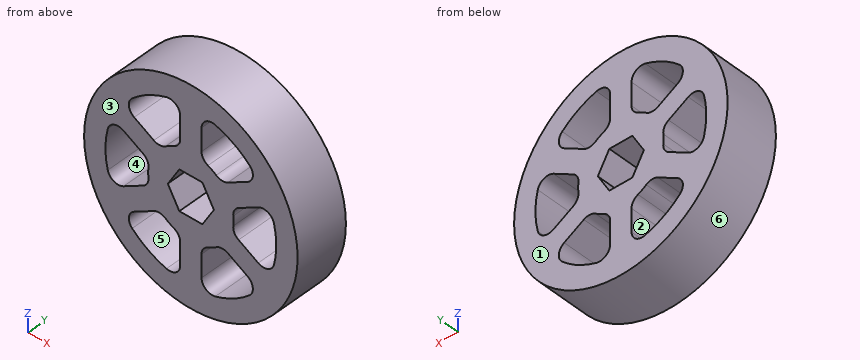
Autodesk Inventor part; units mm, degrees
ref_plane "YZ Plane" through (0, 0, 0) normal (1, 0, 0) x (0, 1, 0)
ref_plane "XZ Plane" through (0, 0, 0) normal (0, 1, 0) x (-1, 0, 0)
ref_plane "XY Plane" through (0, 0, 0) normal (0, 0, 1) x (1, 0, 0)
sketch "Sketch1" plane through (0, 0, 0) normal (0, 1, 0) x (-1, 0, 0)
  circle A0 centre (0, 0) radius 25.4
  line L0 (-2.7424, 4.75) -> (2.7424, 4.75)
  line L1 (2.7424, 4.75) -> (5.4848, 0)
  line L2 (5.4848, 0) -> (2.7424, -4.75)
  line L3 (2.7424, -4.75) -> (-2.7424, -4.75)
  line L4 (-2.7424, -4.75) -> (-5.4848, 0)
  line L5 (-5.4848, 0) -> (-2.7424, 4.75)
  line L6 (2.54, -9.8374) -> (2.54, -20.1606)
  line L7 (-2.54, -9.8374) -> (-2.54, -20.1606)
  line L8 (0, -11.1125) -> (0, -22.225) construction
  line L9 (9.7894, -2.719) -> (18.7296, -7.8806)
  line L10 (7.2494, -7.1184) -> (16.1896, -12.28)
  line L11 (7.2494, 7.1184) -> (16.1896, 12.28)
  line L12 (9.7894, 2.719) -> (18.7296, 7.8806)
  line L13 (-2.54, 9.8374) -> (-2.54, 20.1606)
  line L14 (2.54, 9.8374) -> (2.54, 20.1606)
  line L15 (-9.7894, 2.719) -> (-18.7296, 7.8806)
  line L16 (-7.2494, 7.1184) -> (-16.1896, 12.28)
  line L17 (-7.2494, -7.1184) -> (-16.1896, -12.28)
  line L18 (-9.7894, -2.719) -> (-18.7296, -7.8806)
  arc A1 (9.7894, -2.719) -> (9.7894, 2.719) centre (0, 0) ccw
  arc A2 (7.2494, 7.1184) -> (2.54, 9.8374) centre (0, 0) ccw
  arc A3 (-2.54, 9.8374) -> (-7.2494, 7.1184) centre (0, 0) ccw
  arc A4 (-9.7894, 2.719) -> (-9.7894, -2.719) centre (0, 0) ccw
  arc A5 (-16.1896, -12.28) -> (-2.54, -20.1606) centre (0, 0) ccw
  arc A6 (2.54, -20.1606) -> (16.1896, -12.28) centre (0, 0) ccw
  arc A7 (18.7296, -7.8806) -> (18.7296, 7.8806) centre (0, 0) ccw
  arc A8 (16.1896, 12.28) -> (2.54, 20.1606) centre (0, 0) ccw
  arc A9 (-2.54, 20.1606) -> (-16.1896, 12.28) centre (0, 0) ccw
  arc A10 (-18.7296, 7.8806) -> (-18.7296, -7.8806) centre (0, 0) ccw
  arc A11 (-7.2494, -7.1184) -> (-2.54, -9.8374) centre (0, 0) ccw
  arc A12 (2.54, -9.8374) -> (7.2494, -7.1184) centre (0, 0) ccw
  dimension "d1" = 9.5
  dimension "d4" = 5.08
  dimension "d7" = 360
  dimension "d9" = 20.32
  dimension "d10" = 10.16
  dimension "d11" = 25.4
extrude "Extrusion1" add sketch "Sketch1" along normal blind 12.7
fillet "Fillet1" radius 2.54 4 edges at (16.1896, 6.35, 12.28) (7.2494, 6.35, 7.1184) (2.54, 6.35, 9.8374) (2.54, 6.35, 20.1606)
pattern_circular "Circular Pattern1" count 6 over 360 about axis through (0, 0, 0) along (0, 1, 0) of "Fillet1"
properties part number "2in mould"
Part model, mm, in its own coordinate system. Face numbers are marked on the shaded views. A direction names the side the tool comes from. Coordinates: 2 decimals unless noted, no trailing zeros. Loops run counter-clockwise (first coordinate to the right, second up) from the corner with the lowest first, then second, coordinate; pieces in that order, holes last. Notation, with made-up numbers: (34.5, 42) -> (47.5, 42) arc R26 cw to (47.5, 67) -> close; hole circle Ø11 at (66, 28). An arc over 180 degrees is marked (long way). Use a Markdown table: item, result. Add a question column.
Item 1: Band-saw the part on D-D on x = -7.5. Write the cut outline in (y, z).
Item 2: Band-saw the part on B-B on z = -5.5. Write the cut outline in (x, y).
Item 3: Pull direction X, two halves, no side cores. Call the marked faces 3, 4, 5 and 6: +X half, -X half, draft (parallel to the pull), parting line (faces both ways), or undercut.
Item 4: Probe probe 1 along Z at (x, y) = (-11, 3.25); probe 2 along X at (y, z) = (2.5, 15); probe 3 along Z at (x, y) = (-11.5, 1). List the from-to ranges inside material, lowest first.
Item 5: Band-saw the part on A-A on x = 0. Write the cut outline in (y, z).
Item 6: Band-saw the part on C-C on y = 3.5. Give the number of separate pieces and of enclosed holes in the cut face, plus the area to 3 significant figures.
Item 7: Flat gauge pins, fed straight in: P1, Ø4.5, axis at x = 0, y = 8.5, coming from the +Z side; P2, Ø2.5, axis at y = 4.5, z = -14.5, coming from the -X side; P3, Ø1.5, axis at y = 7.5, z = 19, coming from the +X side. Where does each tip first touch, or does it go through?
Item 8: Which spindle directions (+Z, -Z, +X, -X, +Y, -Y) get a long thin tool onto all of the face, cutting with end or side? Do the marked faces 1 and 2. Say none if no direction does.
Geometry says:
| question | item | result |
|---|---|---|
| 1 | outline | (0, -24.27) -> (12.7, -24.27) -> (12.7, -18.89) -> (0, -18.89) -> close; (0, -7.68) -> (12.7, -7.68) -> (12.7, 7.68) -> (0, 7.68) -> close; (0, 18.89) -> (12.7, 18.89) -> (12.7, 24.27) -> (0, 24.27) -> close |
| 2 | outline | (-24.8, 0) -> (-19.43, 0) -> (-19.43, 12.7) -> (-24.8, 12.7) -> close; (-14.61, 0) -> (14.61, 0) -> (14.61, 12.7) -> (-14.61, 12.7) -> close; (19.43, 0) -> (24.8, 0) -> (24.8, 12.7) -> (19.43, 12.7) -> close |
| 3 | face 3 | draft |
| 3 | face 4 | undercut |
| 3 | face 5 | undercut |
| 3 | face 6 | parting line |
| 4 | probe 1 | -22.89 to -17.09, -9.28 to -3.38, 3.38 to 9.28, 17.09 to 22.89 |
| 4 | probe 2 | -20.5 to -13.71, -2.54 to 2.54, 13.71 to 20.5 |
| 4 | probe 3 | -22.65 to -16.75, -9.57 to -3.71, 3.71 to 9.57, 16.75 to 22.65 |
| 5 | outline | (0, -25.4) -> (12.7, -25.4) -> (12.7, -4.75) -> (0, -4.75) -> close; (0, 4.75) -> (12.7, 4.75) -> (12.7, 25.4) -> (0, 25.4) -> close |
| 6 | separate pieces | 1 |
| 6 | enclosed holes | 7 |
| 6 | area | 1,320 mm² |
| 7 | P1 | z = 25.4 |
| 7 | P2 | x = -21.67 |
| 7 | P3 | x = 17.67 |
| 8 | face 1 | +Z, -Z, +X, -X, +Y |
| 8 | face 2 | +Y, -Y |
